Part model, mm, in its own coordinate system. A direction names the side the tool comes from. Give positions to 0.01 mm unless a question says otherwise; leave off trailing zeros. Write each loop counter-clockwise with the first axis right and the second up, starting at its lowest first coordinate (ties: lowest second). Pieces come first, ordered by that corner, then holes. Notation, with made-up numbers: (46, 21) - (86, 21) arc R25 cw to (86, 45) - close; hole circle Ø2 at (-11, 27). An arc over 180 degrees is marked (long way). Answer as a JSON object with one key per item and string values. Group by question number.
```python
from build123d import *

# Parameters (mm, degrees)
SKETCH1_R           = 1.5875
SKETCH1_W           = 6.35
SKETCH1_H           = 25.4
BOSS_EXTRUDE1_DEPTH = 6.35


with BuildPart() as part:
    # Sketch1 → Boss-Extrude1 (new body)
    with BuildSketch(Plane.XY):
        Polygon((-80.70648923, -31.56367818), (-80.70648923, -21.997051347), (-77.53148923, -21.997051347), (-77.53148923, -23.749651347), (-74.99148923, -23.749651347), (-74.99148923, -21.997051347), (-73.72148923, -21.997051347), (-73.72148923, -18.949191991), (-74.99148923, -18.949191991), (-74.99148923, -17.196591991), (-77.53148923, -17.196591991), (-77.53148923, -18.949191991), (-80.70648923, -18.949191991), (-80.70648923, -9.28787818), (-87.05648923, -9.28787818), (-87.05648923, 16.11212182), (-80.70648923, 16.11212182), (71.69351077, 16.11212182), (71.69351077, -56.96367818), (-80.70648923, -56.96367818), (-87.05648923, -56.96367818), (-87.05648923, -31.56367818), align=None)
        with Locations((-26.73148923, 4.19317182)):
            Circle(SKETCH1_R, mode=Mode.SUBTRACT)
        with Locations((-26.73148923, -45.04472818)):
            Circle(SKETCH1_R, mode=Mode.SUBTRACT)
        with Locations((55.81851077, 4.19317182)):
            Circle(SKETCH1_R, mode=Mode.SUBTRACT)
        with Locations((55.81851077, -45.04472818)):
            Circle(SKETCH1_R, mode=Mode.SUBTRACT)
        with Locations((-53.71898923, 12.93712182)):
            Circle(SKETCH1_R, mode=Mode.SUBTRACT)
        with Locations((14.54351077, 12.93712182)):
            Circle(SKETCH1_R, mode=Mode.SUBTRACT)
        with Locations((-53.64679782, -53.840086503)):
            Circle(SKETCH1_R, mode=Mode.SUBTRACT)
        with Locations((14.615542619, -53.692492422)):
            Circle(SKETCH1_R, mode=Mode.SUBTRACT)
        with Locations((-26.73148923, -20.42577818)):
            Rectangle(SKETCH1_W, SKETCH1_H, mode=Mode.SUBTRACT)
        with Locations((55.81851077, -20.42577818)):
            Rectangle(SKETCH1_W, SKETCH1_H, mode=Mode.SUBTRACT)
        with Locations((14.54351077, -20.42577818)):
            Rectangle(SKETCH1_W, SKETCH1_H, mode=Mode.SUBTRACT)
    extrude(amount=BOSS_EXTRUDE1_DEPTH)


solid = part.part
```
1) Probe line 1 (Y direction, x = 56, z = 0.75); line 2 (X direction, y = -18, z = 2.75); line 3 (X direction, y = -28.5, z = 0.5). List the from-to ranges inside material, lowest first.
2) Band-saw the part on A-A (y = -27.5). List the corners of the cut face in (x, z), plus the area to 3 significant figures.
3) Mould opens along Y. For faces 1 (the flat face through (-7, -20, 0)), 2 (the flat face through (-9, -56.964, 3)), 3 (the flat face through (56, -7.726, 3)), 4 (the flat face through (-7, 16.112, 3)) say: pulls with the +Y half, pulls with the -Y half, needs draft (parallel to the pull), parting line crosses it, or undercut.
4) Drop flat-ended pins along their axis: P1, Ø1.4, axis at y = -22.5, z = 3, coming from the -X side; P2, Ø1.9, axis at x = -53.72, y = 12.94, coming from the -Z side; P3, Ø5, axis at x = 14.54, y = 12.94, coming from the +Z side. Give the stop position or say it passes through.
5) Which spindle directions (+Z, -Z, +X, -X, +Y, -Y) get a long thin tool onto all of the face, cutting with end or side? Do faces 5 (the flat face through (-80.706, -27, 3)), 6 (the flat face through (71.694, -20, 3)), 7 (the flat face through (11.369, -21, 3)). Say none if no direction does.
6) Band-saw the part on B-B (z = 4). State how many separate pieces and enclosed holes the cut face has, plus the area to 3 significant figures.
Verdict:
{
 "1": {"line 1": "-56.96 to -46.62, -43.47 to -33.13, -7.73 to 2.62, 5.77 to 16.11", "line 2": "-80.71 to -77.53, -74.99 to -29.91, -23.56 to 11.37, 17.72 to 52.64, 58.99 to 71.69", "line 3": "-80.71 to -29.91, -23.56 to 11.37, 17.72 to 52.64, 58.99 to 71.69"},
 "2": {"outline": "(-80.71, 0) - (-29.91, 0) - (-29.91, 6.35) - (-80.71, 6.35) - close; (-23.56, 0) - (11.37, 0) - (11.37, 6.35) - (-23.56, 6.35) - close; (17.72, 0) - (52.64, 0) - (52.64, 6.35) - (17.72, 6.35) - close; (58.99, 0) - (71.69, 0) - (71.69, 6.35) - (58.99, 6.35) - close", "area": "847 mm2"},
 "3": {"face 1": "needs draft", "face 2": "pulls with the -Y half", "face 3": "undercut", "face 4": "pulls with the +Y half"},
 "4": {"P1": "x = -80.71", "P2": "through", "P3": "z = 6.35"},
 "5": {"face 5": "+Z, -Z, -X", "face 6": "+Z, -Z, +X, +Y, -Y", "face 7": "+Z, -Z"},
 "6": {"separate pieces": "1", "enclosed holes": "11", "area": "10,900 mm2"}
}
